```python
from build123d import *

# Parameters (mm, degrees)
CIRCLE003_AS_DRAWN_R                    = 9
EXTRUDE012_DEPTH                        = 10
EXTRUDE012_ONTO_CIRCLE003_ROLL_ANGLE    = 90
RECTANGLE006_AS_DRAWN_W                 = 15.8
RECTANGLE006_AS_DRAWN_H                 = 20.5
EXTRUDE011_DEPTH                        = 10
EXTRUDE011_ONTO_RECTANGLE006_ROLL_ANGLE = 90


with BuildPart() as extrude012:
    # Circle003 as drawn → Extrude012 (new)
    with BuildSketch(Plane.XY):
        Circle(CIRCLE003_AS_DRAWN_R)
    extrude(amount=-EXTRUDE012_DEPTH)


with BuildPart() as extrude012_1:
    # Extrude012 onto Circle003 roll: moved
    add(extrude012.part.rotate(Axis((0, 0, 0), (1, 0, 0)), EXTRUDE012_ONTO_CIRCLE003_ROLL_ANGLE))


with BuildPart() as extrude012_2:
    # Extrude012 onto Circle003 placement: moved
    add(extrude012_1.part.moved(Location((-26.421617, -16.969141, -4.904319))))


with BuildPart() as corpomotor:
    # Rectangle006 as drawn → Extrude011 (new)
    with BuildSketch(Plane.XY):
        with Locations((7.9, 10.25)):
            Rectangle(RECTANGLE006_AS_DRAWN_W, RECTANGLE006_AS_DRAWN_H)
    extrude(amount=-EXTRUDE011_DEPTH)


with BuildPart() as corpomotor_1:
    # Extrude011 onto Rectangle006 roll: moved
    add(corpomotor.part.rotate(Axis((0, 0, 0), (1, 0, 0)), EXTRUDE011_ONTO_RECTANGLE006_ROLL_ANGLE))


with BuildPart() as corpomotor_2:
    # Extrude011 onto Rectangle006 placement: moved
    add(corpomotor_1.part.moved(Location((-34.321617, -16.969141, -15.154319))))

    # Common002: intersect Extrude012
    add(extrude012_2.part, mode=Mode.INTERSECT)


with BuildPart() as corpomotor_3:
    # Common002 placement: moved
    add(corpomotor_2.part.moved(Location((36.106213, 66.825929, 15.967406))))


solid = corpomotor_3.part
```
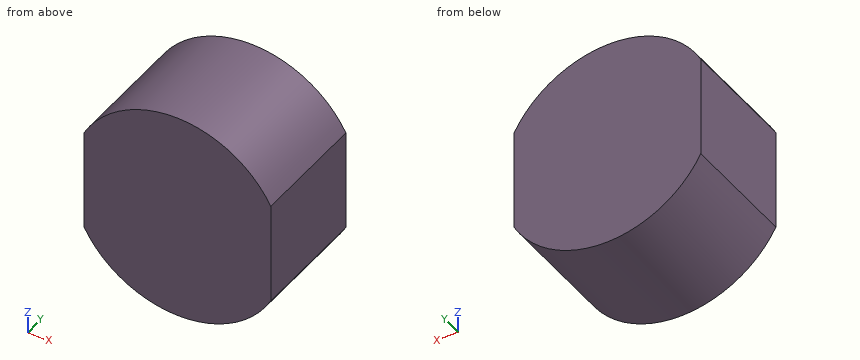
Verification items for the finished model (mm, model axes). Round coordinates to 2 decimals unless told otherwise and drop trailing zeros. Write each loop counter-clockwise with the first axis right and the second up, starting at its lowest first coordinate (ties: lowest second). Pieces come first, ordered by that corner, then holes. Notation, with made-up numbers: (66.5, -30) - (99.5, -30) arc R25 ccw to (99.5, -8) - close; hole circle Ø1 at (63, -35). An arc over 180 degrees is marked (long way). Answer as a JSON object with one key per item and string values. Group by question number.
Q1. Section check B-B, the plane x = 15.75. Enter the section's corners in (y, z), plus the area to 3 significant figures.
Q2. Section check A-A, the plane y = 55.5. Enter the section's corners in (x, z), plus the area to 3 significant figures.
Q3. Go/stop test with flat-tipped pins: pin 1 Ø4 at (x, y) = (7.5, 59) entering from -Z (3 decimals); pin 2 Ø3 at (x, y) = (6.5, 54) entering from +Z; pin 3 Ø1.5 at (x, y) = (11, 51.5) entering from +Z. Record where each tip stops, or that it passes through.
Q4. Thickness scan on line 1 (Z direction, x = 16.5, y = 53.25); line 2 (X direction, y = 55, z = 5.5); line 3 (Z direction, x = 9.5, y = 51.75). Record the ranges inside material, lowest first.
Found:
{
 "1": {"outline": "(49.86, 4.41) - (59.86, 4.41) - (59.86, 17.71) - (49.86, 17.71) - close", "area": "133 mm^2"},
 "2": {"outline": "(1.78, 6.75) arc R9 ccw to (17.58, 6.75) - (17.58, 15.37) arc R9 ccw to (1.78, 15.37) - close", "area": "242 mm^2"},
 "3": {"pin 1": "stops at z = 2.065", "pin 2": "stops at z = 19.9", "pin 3": "stops at z = 20.05"},
 "4": {"line 1": "z = 5.19 to 16.94", "line 2": "x = 2.61 to 16.76", "line 3": "z = 2.06 to 20.06"}
}
